from build123d import *

# Parameters (mm, degrees)
F1_DEPTH = 88.9
F3_R     = 12.7635
F4_DEPTH = 5
F5_D     = 2.9464
F6_D     = 4


with BuildPart() as f1:
    # F0 (on Top) → F1 (new body)
    with BuildSketch(Plane.XY):
        with BuildLine():
            ThreePointArc((-8.3979817921, -11.5588303071), (-8.0866479786, -11.7787427479), (-7.7695585406, -11.9902717373))
            Line((-7.7695585406, -11.9902717373), (-6.8723442619, -10.7553622252))
            ThreePointArc((-6.8723442619, -10.7553622252), (-6.1315481839, 11.194241784), (12.7635, 0))
            ThreePointArc((12.7635, 0), (11.194241784, -6.1315481839), (6.8723442619, -10.7553622252))
            Line((6.8723442619, -10.7553622252), (7.7695585406, -11.9902717373))
            ThreePointArc((7.7695585406, -11.9902717373), (8.0866479786, -11.7787427479), (8.3979817921, -11.5588303071))
            ThreePointArc((8.3979817921, -11.5588303071), (8.7033383912, -11.3306909365), (9.00250044, -11.0944870128))
            ThreePointArc((9.00250044, -11.0944870128), (12.8987573294, -6.1444866023), (14.2875, 0))
            ThreePointArc((14.2875, 0), (14.1661979921, 1.8578188013), (13.8043516957, 3.6840915448))
            ThreePointArc((13.8043516957, 3.6840915448), (13.701161697, 4.0510275736), (13.5882199766, 4.4150803071))
            ThreePointArc((13.5882199766, 4.4150803071), (13.46560692, 4.7759906331), (13.3334097963, 5.1335016756))
            ThreePointArc((13.3334097963, 5.1335016756), (8.3979817921, 11.5588303071), (0.762, 14.2671655296))
            ThreePointArc((0.762, 14.2671655296), (0.3811356355, 14.2824154777), (0, 14.2875))
            ThreePointArc((0, 14.2875), (-0.3811356355, 14.2824154777), (-0.762, 14.2671655296))
            ThreePointArc((-0.762, 14.2671655296), (-8.3979817921, 11.5588303071), (-13.3334097963, 5.1335016756))
            ThreePointArc((-13.3334097963, 5.1335016756), (-13.4656069199, 4.7759906331), (-13.5882199766, 4.4150803071))
            ThreePointArc((-13.5882199766, 4.4150803071), (-13.701161697, 4.0510275736), (-13.8043516957, 3.6840915448))
            ThreePointArc((-13.8043516957, 3.6840915448), (-13.5882199766, -4.4150803071), (-9.00250044, -11.0944870128))
            ThreePointArc((-9.00250044, -11.0944870128), (-8.7033383912, -11.3306909365), (-8.3979817921, -11.5588303071))
        make_face()
        with BuildLine():
            ThreePointArc((0, 36.576), (-0.3810206745, 36.5740153558), (-0.762, 36.5680616385))
            Line((-0.762, 36.5680616385), (-0.762, 14.2671655296))
            ThreePointArc((-0.762, 14.2671655296), (-0.3811356355, 14.2824154777), (0, 14.2875))
            Line((0, 14.2875), (0, 36.576))
        make_face()
        with BuildLine():
            ThreePointArc((0.762, 36.5680616385), (0.3810206745, 36.5740153558), (0, 36.576))
            Line((0, 36.576), (0, 14.2875))
            ThreePointArc((0, 14.2875), (0.3811356355, 14.2824154777), (0.762, 14.2671655296))
            Line((0.762, 14.2671655296), (0.762, 36.5680616385))
        make_face()
        with BuildLine():
            Line((13.5882199766, 4.4150803071), (34.78584314, 11.3026055863))
            ThreePointArc((34.78584314, 11.3026055863), (34.6662137676, 11.6643644928), (34.5428223599, 12.0248575631))
            Line((34.5428223599, 12.0248575631), (13.3334097963, 5.1335016756))
            ThreePointArc((13.3334097963, 5.1335016756), (13.46560692, 4.7759906331), (13.5882199766, 4.4150803071))
        make_face()
        with BuildLine():
            Line((13.8043516957, 3.6840915448), (35.0137642593, 10.5754474322))
            ThreePointArc((35.0137642593, 10.5754474322), (34.9016974948, 10.9396201021), (34.78584314, 11.3026055863))
            Line((34.78584314, 11.3026055863), (13.5882199766, 4.4150803071))
            ThreePointArc((13.5882199766, 4.4150803071), (13.701161697, 4.0510275736), (13.8043516957, 3.6840915448))
        make_face()
        with BuildLine():
            ThreePointArc((-34.5428223599, 12.0248575631), (-34.6662137676, 11.6643644928), (-34.78584314, 11.3026055863))
            Line((-34.78584314, 11.3026055863), (-13.5882199766, 4.4150803071))
            ThreePointArc((-13.5882199766, 4.4150803071), (-13.4656069199, 4.7759906331), (-13.3334097963, 5.1335016756))
            Line((-13.3334097963, 5.1335016756), (-34.5428223599, 12.0248575631))
        make_face()
        with BuildLine():
            ThreePointArc((-34.78584314, 11.3026055863), (-34.9016974948, 10.9396201021), (-35.0137642593, 10.5754474322))
            Line((-35.0137642593, 10.5754474322), (-13.8043516957, 3.6840915448))
            ThreePointArc((-13.8043516957, 3.6840915448), (-13.701161697, 4.0510275736), (-13.5882199766, 4.4150803071))
            Line((-13.5882199766, 4.4150803071), (-34.78584314, 11.3026055863))
        make_face()
        with BuildLine():
            ThreePointArc((21.773667791, -31.2652745218), (33.7726719615, -17.6356635424), (38.1, 0))
            ThreePointArc((38.1, 0), (-17.6356635424, 33.7726719615), (-21.773667791, -31.2652745218))
            Line((-21.773667791, -31.2652745218), (-20.8776963863, -30.0320756792))
            ThreePointArc((-20.8776963863, -30.0320756792), (-21.1894146424, -29.8129583087), (-21.4988333878, -29.5906055863))
            ThreePointArc((-21.4988333878, -29.5906055863), (-21.8059190441, -29.3650416421), (-22.1106382858, -29.1362909547))
            ThreePointArc((-22.1106382858, -29.1362909547), (-34.78584314, -11.3026055863), (-35.0137642593, 10.5754474322))
            ThreePointArc((-35.0137642593, 10.5754474322), (-34.9016974948, 10.9396201021), (-34.78584314, 11.3026055863))
            ThreePointArc((-34.78584314, 11.3026055863), (-34.6662137676, 11.6643644928), (-34.5428223599, 12.0248575631))
            ThreePointArc((-34.5428223599, 12.0248575631), (-21.4988333878, 29.5906055863), (-0.762, 36.5680616385))
            ThreePointArc((-0.762, 36.5680616385), (-0.3810206745, 36.5740153558), (0, 36.576))
            ThreePointArc((0, 36.576), (0.3810206745, 36.5740153558), (0.762, 36.5680616385))
            ThreePointArc((0.762, 36.5680616385), (21.4988333878, 29.5906055863), (34.5428223599, 12.0248575631))
            ThreePointArc((34.5428223599, 12.0248575631), (34.6662137676, 11.6643644928), (34.78584314, 11.3026055863))
            ThreePointArc((34.78584314, 11.3026055863), (34.9016974948, 10.9396201021), (35.0137642593, 10.5754474322))
            ThreePointArc((35.0137642593, 10.5754474322), (36.183333301, 5.3451068488), (36.576, 0))
            ThreePointArc((36.576, 0), (32.7606660642, -16.264763602), (22.1106382858, -29.1362909547))
            ThreePointArc((22.1106382858, -29.1362909547), (21.8059190441, -29.3650416421), (21.4988333878, -29.5906055863))
            ThreePointArc((21.4988333878, -29.5906055863), (21.1894146424, -29.8129583087), (20.8776963863, -30.0320756792))
            Line((20.8776963863, -30.0320756792), (21.773667791, -31.2652745218))
        make_face()
        with BuildLine():
            Line((7.7695585406, -11.9902717373), (20.8776963863, -30.0320756792))
            ThreePointArc((20.8776963863, -30.0320756792), (21.1894146424, -29.8129583087), (21.4988333878, -29.5906055863))
            Line((21.4988333878, -29.5906055863), (8.3979817921, -11.5588303071))
            ThreePointArc((8.3979817921, -11.5588303071), (8.0866479786, -11.7787427479), (7.7695585406, -11.9902717373))
        make_face()
        with BuildLine():
            Line((8.3979817921, -11.5588303071), (21.4988333878, -29.5906055863))
            ThreePointArc((21.4988333878, -29.5906055863), (21.8059190441, -29.3650416421), (22.1106382858, -29.1362909547))
            Line((22.1106382858, -29.1362909547), (9.00250044, -11.0944870128))
            ThreePointArc((9.00250044, -11.0944870128), (8.7033383912, -11.3306909365), (8.3979817921, -11.5588303071))
        make_face()
        with BuildLine():
            ThreePointArc((-21.4988333878, -29.5906055863), (-21.1894146424, -29.8129583087), (-20.8776963863, -30.0320756792))
            Line((-20.8776963863, -30.0320756792), (-7.7695585406, -11.9902717373))
            ThreePointArc((-7.7695585406, -11.9902717373), (-8.0866479786, -11.7787427479), (-8.3979817921, -11.5588303071))
            Line((-8.3979817921, -11.5588303071), (-21.4988333878, -29.5906055863))
        make_face()
        with BuildLine():
            ThreePointArc((-22.1106382858, -29.1362909547), (-21.8059190441, -29.3650416421), (-21.4988333878, -29.5906055863))
            Line((-21.4988333878, -29.5906055863), (-8.3979817921, -11.5588303071))
            ThreePointArc((-8.3979817921, -11.5588303071), (-8.7033383912, -11.3306909365), (-9.00250044, -11.0944870128))
            Line((-9.00250044, -11.0944870128), (-22.1106382858, -29.1362909547))
        make_face()
    extrude(amount=F1_DEPTH)

    # F3 (on offset) → F4 (join)
    with BuildSketch(Plane.XY.offset(10)):
        Circle(F3_R)
    extrude(amount=F4_DEPTH)

    # F5 (through all)
    with Locations(Plane(origin=(0, 0, 10), x_dir=(1, 0, 0), z_dir=(0, 0, -1))):
        with Locations((0, -6.35), (6.35, 0), (0, 6.35), (-6.35, 0)):
            Hole(F5_D / 2)

    # F6 (through all)
    with Locations(Plane(origin=(0, 0, 10), x_dir=(1, 0, 0), z_dir=(0, 0, -1))):
        with Locations((0, 0)):
            Hole(F6_D / 2)


solid = f1.part
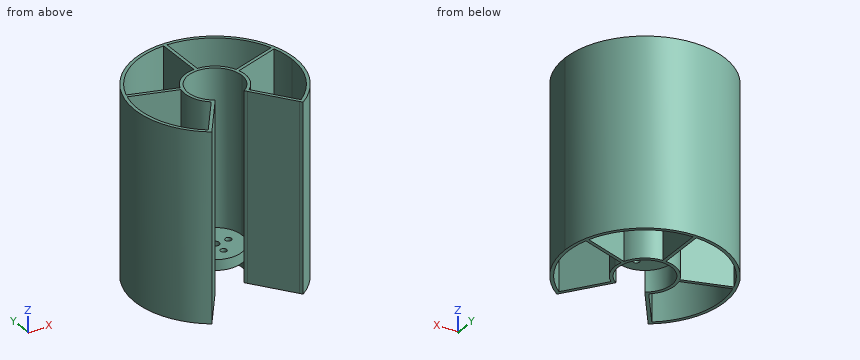
Verification items for the finished model (mm, model axes). Coordinates: 2 decimals unless noted, no trailing zeros. Write each loop counter-clockwise with the first axis right and the second up, starting at its lowest first coordinate (ties: lowest second). Pieces come first, ordered by that corner, then holes. Notation, with made-up numbers: (52, 5) - (107, 5) arc R24 ccw to (107, 19) - close; hole circle Ø7 at (-20.75, 57). An arc over 180 degrees is marked (long way). Answer as a JSON object with one key per item and string values.
(1) Cross-section at A-A on y = 33. Record the cut outline in (x, z), plus the area to 3 significant figures.
Report:
{"outline": "(-19.04, 0) - (-15.77, 0) - (-15.77, 88.9) - (-19.04, 88.9) - close; (-0.76, 0) - (0.76, 0) - (0.76, 88.9) - (-0.76, 88.9) - close; (15.77, 0) - (19.04, 0) - (19.04, 88.9) - (15.77, 88.9) - close", "area": "717 mm^2"}
(2) Cross-section at C-C on x = -30.5. Record the cut outline in (y, z).
Report:
{"outline": "(-22.83, 0) - (-20.19, 0) - (-20.19, 88.9) - (-22.83, 88.9) - close; (9.11, 0) - (10.71, 0) - (10.71, 88.9) - (9.11, 88.9) - close; (20.19, 0) - (22.83, 0) - (22.83, 88.9) - (20.19, 88.9) - close"}
(3) Cross-section at D-D on y = -25.5. Record the cut outline in (x, z), plus the area to 3 significant figures.
Report:
{"outline": "(-28.31, 0) - (-26.22, 0) - (-26.22, 88.9) - (-28.31, 88.9) - close; (-19.47, 0) - (-17.58, 0) - (-17.58, 88.9) - (-19.47, 88.9) - close; (17.58, 0) - (19.47, 0) - (19.47, 88.9) - (17.58, 88.9) - close; (26.22, 0) - (28.31, 0) - (28.31, 88.9) - (26.22, 88.9) - close", "area": "706 mm^2"}
(4) Thickness scan on line 1 along Y through (x, z) = (-27, 84); line 2 along X through (y, z) = (-6.35, 11.5); line 3 along Y through (x, z) = (-22, 18.5). Record the ranges inside material, lowest first.
Report:
{"line 1": "-26.88 to -24.67, 7.97 to 9.57, 24.67 to 26.88", "line 2": "-37.57 to -36.02, -12.8 to -1.47, 1.47 to 12.8, 36.02 to 37.57", "line 3": "-31.11 to -28.98, 6.35 to 7.95, 29.22 to 31.11"}
(5) Gauge pin test, flat ends, axial feed: pin 1 Ø5 at (x, y) = (0, 0) entering from +Z; pin 2 Ø4 at (x, y) = (24, 10.5) entering from -Z; pin 3 Ø7.5 at (x, y) = (3.5, 2.5) entering from -Z; pin 4 Ø3 at (y, z) = (-4.5, 44) entering from -X. Record the tip position at first contact, or that the pin passes through.
Report:
{"pin 1": "z = 15", "pin 2": "z = 0", "pin 3": "z = 10", "pin 4": "x = -37.98"}
(6) Cross-section at B-B on z = 22. Record the cut outline in (x, y) (1 decimal).
Report:
{"outline": "(-21.8, -31.3) - (-6.9, -10.8) arc R12.8 cw (long way) to (6.9, -10.8) - (21.8, -31.3) arc R38.1 ccw (long way) to start; hole (-35, 10.6) arc R36.6 ccw to (-22.1, -29.1) - (-9, -11.1) arc R14.3 cw to (-13.8, 3.7) - close; hole (-34.5, 12) - (-13.3, 5.1) arc R14.3 cw to (-0.8, 14.3) - (-0.8, 36.6) arc R36.6 ccw to start; hole (0.8, 14.3) arc R14.3 cw to (13.3, 5.1) - (34.5, 12) arc R36.6 ccw to (0.8, 36.6) - close; hole (9, -11.1) - (22.1, -29.1) arc R36.6 ccw to (35, 10.6) - (13.8, 3.7) arc R14.3 cw to start"}
